Geometry: final body of the model. Coordinates: model frame, mm. Face numbers are marked on the shaded views. Round coordinates to 2 decimals unless told otherwise and drop trailing zeros. Loops run counter-clockwise (first coordinate to the right, second up) from the corner with the lowest first, then second, coordinate; pieces in that order, holes last. Notation, with made-up numbers: M 11.5,0.25 L 19.5,0.25 A18 cw 19.5,35.25 Z; hole C 87,82.5 d4. An arc over 180 degrees is marked long. Answer as a JSON object with one key per item and string values.
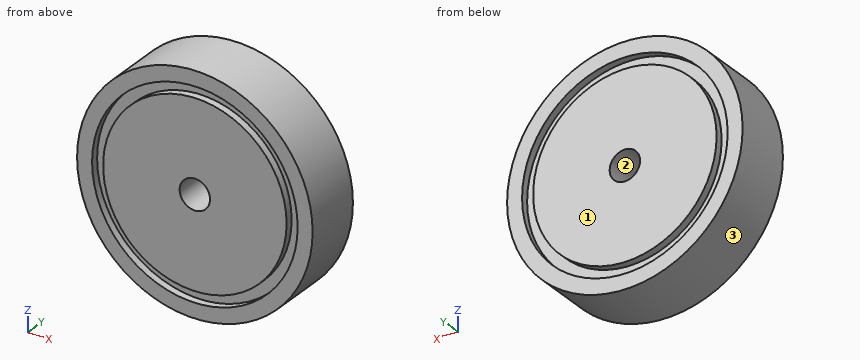
from build123d import *

# Parameters (mm, degrees)
F0_R     = 77.5
F1_DEPTH = 20
F2_R     = 67.6447
F2_R_2   = 60.383238
F3_DEPTH = 5
F4_R     = 67.6447
F4_R_2   = 60.383238
F5_DEPTH = 5
F6_R     = 10
F7_DEPTH = 40.001


with BuildPart() as f1:
    # F0 (on Front) → F1 (new body, symmetric)
    with BuildSketch(Plane.XZ):
        Circle(F0_R)
    extrude(amount=F1_DEPTH, both=True)

    # F2 (on face) → F3 (cut)
    with BuildSketch(Plane(origin=(0, 20, 0), x_dir=(-1, 0, 0), z_dir=(0, 1, 0))):
        Circle(F2_R)
        Circle(F2_R_2, mode=Mode.SUBTRACT)
    extrude(amount=-F3_DEPTH, mode=Mode.SUBTRACT)

    # F4 (on face) → F5 (cut)
    with BuildSketch(Plane.XZ.offset(20)):
        Circle(F4_R)
        Circle(F4_R_2, mode=Mode.SUBTRACT)
    extrude(amount=-F5_DEPTH, mode=Mode.SUBTRACT)

    # F6 (on face) → F7 (cut, through all)
    with BuildSketch(Plane.XZ.offset(20)):
        Circle(F6_R)
    extrude(amount=-F7_DEPTH, mode=Mode.SUBTRACT)


solid = f1.part
1) Ray query, line 1 (X direction, y = 16.5, z = 26); line 2 (Y direction, x = 47.5, z = -40.5); line 3 (X direction, y = 4, z = -64.5). Return the intervals inside material, ascending.
Results:
{"line 1": "-73.01 to -62.45, -54.5 to 54.5, 62.45 to 73.01", "line 2": "-15 to 15", "line 3": "-42.97 to 42.97"}
2) Section query B-B (z = 0). Return the cut outline in (x, y), and give its area (3 significant figures).
Results:
{"outline": "M -77.5,-20 L -67.64,-20 L -67.64,-15 L -60.38,-15 L -60.38,-20 L -10,-20 L -10,20 L -60.38,20 L -60.38,15 L -67.64,15 L -67.64,20 L -77.5,20 Z; M 10,-20 L 60.38,-20 L 60.38,-15 L 67.64,-15 L 67.64,-20 L 77.5,-20 L 77.5,20 L 67.64,20 L 67.64,15 L 60.38,15 L 60.38,20 L 10,20 Z", "area": "5,250 mm2"}
3) Section query C-C (y = 12). Return the cut outline in (x, z).
Results:
{"outline": "C 0,0 d155; hole C 0,0 d20"}
4) Section query A-A (x = 0). Return the cut outline in (y, z).
Results:
{"outline": "M -20,-77.5 L 20,-77.5 L 20,-67.64 L 15,-67.64 L 15,-60.38 L 20,-60.38 L 20,-10 L -20,-10 L -20,-60.38 L -15,-60.38 L -15,-67.64 L -20,-67.64 Z; M -20,10 L 20,10 L 20,60.38 L 15,60.38 L 15,67.64 L 20,67.64 L 20,77.5 L -20,77.5 L -20,67.64 L -15,67.64 L -15,60.38 L -20,60.38 Z"}
5) Pull-direction query (Z, two-part tool) for the marked faces 1, 2 and 3; classes: +Z half, -Z half, draft (parallel to the pull), parting line (faces both ways), or undercut.
Results:
{"face 1": "draft", "face 2": "undercut", "face 3": "parting line"}
6) Pin query (flat end, axial travel): P1, Ø5, axis at x = 51, y = -5.5, coming from the +Z side; P2, Ø12, axis at x = 12, y = 7.5, coming from the -Z side; P3, Ø6, axis at y = -0.5, z = 57.5, coming from the +X side. Return the tip coordinate at first contact, or that it passes through.
Results:
{"P1": "z = 60.45", "P2": "z = -77.27", "P3": "x = 55.1"}
7) Section query D-D (x = -58). Return the cut outline in (y, z), and give its area (3 significant figures).
Results:
{"outline": "M -20,-51.4 L 20,-51.4 L 20,-34.81 L 15,-34.81 L 15,-16.8 L 20,-16.8 L 20,16.8 L 15,16.8 L 15,34.81 L 20,34.81 L 20,51.4 L -20,51.4 L -20,34.81 L -15,34.81 L -15,16.8 L -20,16.8 L -20,-16.8 L -15,-16.8 L -15,-34.81 L -20,-34.81 Z", "area": "3,750 mm2"}
